from build123d import *
from OCP.BRepFilletAPI import BRepFilletAPI_MakeChamfer

# Parameters (mm, degrees)
SKETCH1_W           = 16
SKETCH1_H           = 16
BOSS_EXTRUDE1_DEPTH = 10
SKETCH2_W           = 8
SKETCH2_H           = 8
CUT_EXTRUDE1_DEPTH  = 1
FILLET4_SIZE        = 2
FILLET4_SIZE2       = 1.2


with BuildPart() as part:
    # Sketch1 → Boss-Extrude1 (new body)
    with BuildSketch(Plane.XY):
        with Locations((8, 8)):
            Rectangle(SKETCH1_W, SKETCH1_H)
    extrude(amount=BOSS_EXTRUDE1_DEPTH)

    # Sketch2 → Cut-Extrude1 (cut)
    with BuildSketch(Plane.XY.offset(10)):
        with Locations((8, 8)):
            Rectangle(SKETCH2_W, SKETCH2_H)
    extrude(amount=-CUT_EXTRUDE1_DEPTH, mode=Mode.SUBTRACT)

    # Fillet4: one chamfer whose edges measure the first distance from different faces: ONE call of the kernel's chamfer builder (chamfer() names one face for all edges)
    fillet4_edges_1 = [part.edges().sort_by_distance(p)[0] for p in [
        (16, 8, 10),
    ]]
    fillet4_side_1 = [part.faces().sort_by_distance(p)[0] for p in [
        (16, 8, 5),
    ]]
    fillet4_edges_2 = [part.edges().sort_by_distance(p)[0] for p in [
        (8, 16, 10),
    ]]
    fillet4_side_2 = [part.faces().sort_by_distance(p)[0] for p in [
        (8, 16, 5),
    ]]
    fillet4_edges_3 = [part.edges().sort_by_distance(p)[0] for p in [
        (0, 8, 10),
    ]]
    fillet4_side_3 = [part.faces().sort_by_distance(p)[0] for p in [
        (0, 8, 5),
    ]]
    fillet4_edges_4 = [part.edges().sort_by_distance(p)[0] for p in [
        (8, 0, 10),
    ]]
    fillet4_side_4 = [part.faces().sort_by_distance(p)[0] for p in [
        (8, 0, 5),
    ]]
    fillet4 = BRepFilletAPI_MakeChamfer(part.part.solid().wrapped)
    for e in fillet4_edges_1:
        fillet4.Add(FILLET4_SIZE, FILLET4_SIZE2, e.wrapped, fillet4_side_1[0].wrapped)  # the first distance lies on this face
    for e in fillet4_edges_2:
        fillet4.Add(FILLET4_SIZE, FILLET4_SIZE2, e.wrapped, fillet4_side_2[0].wrapped)  # the first distance lies on this face
    for e in fillet4_edges_3:
        fillet4.Add(FILLET4_SIZE, FILLET4_SIZE2, e.wrapped, fillet4_side_3[0].wrapped)  # the first distance lies on this face
    for e in fillet4_edges_4:
        fillet4.Add(FILLET4_SIZE, FILLET4_SIZE2, e.wrapped, fillet4_side_4[0].wrapped)  # the first distance lies on this face
    add(Compound.cast(fillet4.Shape()), mode=Mode.REPLACE)


solid = part.part
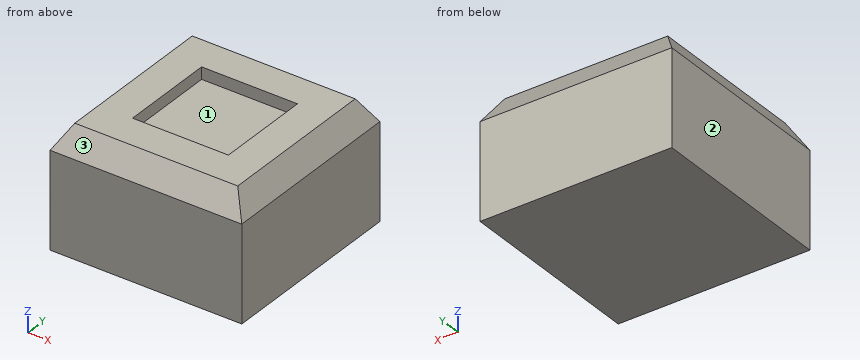
Build history of the part. All positions in model axes, mm. Face numbers are marked on the shaded views. Coordinates: 2 decimals unless noted, no trailing zeros. Order: outer loops, then holes, each group sorted by start corner. A loop starts at its lowest first (then second) coordinate and runs counter-clockwise, first axis right, second up. Notation, with made-up numbers: (77.5, 53) - (86.5, 53) arc R20 ccw to (86.5, 79) - close; hole circle Ø11 at (36, -25). An arc over 180 degrees is marked (long way). Put each result on its own line as item: value.
1. Probe line 1 along Z through (x, y) = (5, 11); line 2 along Y through (x, z) = (8.5, 9.75); line 3 along Y through (x, z) = (1.5, 8.5). List the from-to ranges inside material, lowest first. Write a range as [from, to].
Answer sheet:
line 1: z = [0, 9]
line 2: y = [1.05, 4], [12, 14.95]
line 3: y = [0.3, 15.7]
2. Saw through at A-A (z = 9.25). Write the cut outline in (x, y), and give its area (3 significant figures).
Answer sheet:
outline: (0.75, 0.75) - (15.25, 0.75) - (15.25, 15.25) - (0.75, 15.25) - close; hole (4, 4) - (12, 4) - (12, 12) - (4, 12) - close
area: 146 mm^2
3. Drop flat-ended pins along their axis: P1, Ø4, axis at x = 8.5, y = 6.5, coming from the +Z side; P2, Ø0.8, axis at x = 7.5, z = 9.5, coming from the -Y side; P3, Ø0.8, axis at y = 6.5, z = 9.5, coming from the -X side. Give the stop position or say it passes through.
Answer sheet:
P1: stops at z = 9
P2: stops at y = 0.66
P3: stops at x = 0.66
4. Saw through at B-B (y = 9.25). Write the cut outline in (x, z), and give its area (3 significant figures).
Answer sheet:
outline: (0, 0) - (16, 0) - (16, 8) - (14.8, 10) - (12, 10) - (12, 9) - (4, 9) - (4, 10) - (1.2, 10) - (0, 8) - close
area: 150 mm^2
5. Pull direction X, two halves, no side cores. Call the marked faces 1, 2 and 3: pulls with the +X half, pulls with the -X half, needs draft (parallel to the pull), parting line crosses it, or undercut.
Answer sheet:
face 1: undercut
face 2: pulls with the -X half
face 3: needs draft
6. Saw through at D-D (y = 3). Write the cut outline in (x, z), and give its area (3 significant figures).
Answer sheet:
outline: (0, 0) - (16, 0) - (16, 8) - (14.8, 10) - (1.2, 10) - (0, 8) - close
area: 158 mm^2
